from build123d import *
from build123d.topology import SkipClean

# Parameters (mm, degrees)
BOSS_EXTRUDE1_DEPTH   = 40
CUT_EXTRUDE4_DEPTH    = 149.681707012
FILLET1_R             = 20
CUT_EXTRUDE2_REACH    = 150.682
SKETCH3_R             = 19
M20_TAPPED_HOLE1_D    = 17.5
SKETCH8_R             = 15
CUT_EXTRUDE3_DEPTH    = 10
M6_TAPPED_HOLE1_D     = 5
M6_TAPPED_HOLE1_DEPTH = 17
M6_TAPPED_HOLE1_TIP   = 1.502151548
F_8_0MM_DOWEL_HOLE1_D = 8
CHAMFER1_SIZE         = 1


with BuildPart() as part:
    # Sketch1 → Boss-Extrude1 (new body)
    with BuildSketch(Plane(origin=(0, 0, 0), x_dir=(1, 0, 0), z_dir=(0, 1, 0))):
        with BuildLine():
            Line((-90, 0), (-90, 39.504902432))
            ThreePointArc((-90, 39.504902432), (-85.182396525, 94.862332258), (-30.561841884, 84.652075111))
            ThreePointArc((-30.561841884, 84.652075111), (0, 90), (30.561841884, 84.652075111))
            ThreePointArc((30.561841884, 84.652075111), (85.182396525, 94.862332258), (90, 39.504902432))
            Line((90, 39.504902432), (90, 0))
            ThreePointArc((90, 0), (0, -90), (-90, 0))
        make_face()
    extrude(amount=BOSS_EXTRUDE1_DEPTH)

    # Sketch2 → Cut-Extrude4 (cut, through all)
    with SkipClean():  # the faces are left unmerged after this step: merging them gives an invalid solid
        with BuildSketch(Plane(origin=(0, 0, 0), x_dir=(1, 0, 0), z_dir=(0, 1, 0))):
            with BuildLine():
                Line((-81.25, 32.524047358), (-62.5, 21.698729811))
                Line((-62.5, 21.698729811), (-62.5, 0))
                ThreePointArc((-62.5, 0), (0, -62.5), (62.5, 0))
                Line((62.5, 0), (62.5, 21.698729811))
                Line((62.5, 21.698729811), (81.25, 32.524047358))
                ThreePointArc((81.25, 32.524047358), (85.886934587, 35.68615872), (90, 39.504902432))
                Line((90, 39.504902432), (90, 0))
                ThreePointArc((90, 0), (0, -90), (-90, 0))
                Line((-90, 0), (-90, 39.504902432))
                ThreePointArc((-90, 39.504902432), (-85.886934587, 35.68615872), (-81.25, 32.524047358))
            make_face()
        extrude(amount=CUT_EXTRUDE4_DEPTH, mode=Mode.SUBTRACT)

    # Fillet1
    fillet1_edges = [part.edges().sort_by_distance(p)[0] for p in [
        (30.561841884, 20, -84.652075111),
        (-30.561841884, 20, -84.652075111),
        (-62.5, 20, -21.698729811),
        (62.5, 20, -21.698729811),
    ]]
    fillet(fillet1_edges, radius=FILLET1_R)

    # Sketch3 → Cut-Extrude2 (cut, up to next)
    with BuildSketch(Plane(origin=(0, 0, 0), x_dir=(1, 0, 0), z_dir=(0, 1, 0)), mode=Mode.PRIVATE) as cut_extrude2_sk1:
        with Locations(Location((-62.5, 65, 0), (0, 0, 270))):
            Circle(SKETCH3_R)
    cut_extrude2_tool1 = extrude(cut_extrude2_sk1.sketch, amount=CUT_EXTRUDE2_REACH, mode=Mode.PRIVATE) & part.part
    # Sketch3 → Cut-Extrude2 (cut, up to next)
    with BuildSketch(Plane(origin=(0, 0, 0), x_dir=(1, 0, 0), z_dir=(0, 1, 0)), mode=Mode.PRIVATE) as cut_extrude2_sk2:
        with Locations(Location((62.5, 65, 0), (0, 0, 270))):
            Circle(SKETCH3_R)
    cut_extrude2_tool2 = extrude(cut_extrude2_sk2.sketch, amount=CUT_EXTRUDE2_REACH, mode=Mode.PRIVATE) & part.part
    add(cut_extrude2_tool1.solids().sort_by_distance((-62.5, 0, -65))[0], mode=Mode.SUBTRACT)
    add(cut_extrude2_tool2.solids().sort_by_distance((62.5, 0, -65))[0], mode=Mode.SUBTRACT)

    # M20 Tapped Hole1 (through all)
    with Locations(Plane(origin=(0, 40, 0), x_dir=(1, 0, 0), z_dir=(0, 1, 0))):
        with Locations((0, 0)):
            Hole(M20_TAPPED_HOLE1_D / 2)

    # Sketch8 → Cut-Extrude3 (cut)
    with SkipClean():  # the faces are left unmerged after this step: merging them gives an invalid solid
        with BuildSketch(Plane.XZ):
            with Locations(Location((0, 0, 0), (0, 0, 270))):
                Circle(SKETCH8_R)
        extrude(amount=-CUT_EXTRUDE3_DEPTH, mode=Mode.SUBTRACT)

    # M6 Tapped Hole1
    with Locations(Plane(origin=(0, 0, 0), x_dir=(-1, 0, 0), z_dir=(0, -1, 0))):
        with Locations((-21.650635095, -12.237722392), (21.650635095, -12.5), (0, 25)):
            Hole(M6_TAPPED_HOLE1_D / 2, depth=M6_TAPPED_HOLE1_DEPTH)
            with Locations((0, 0, -(M6_TAPPED_HOLE1_DEPTH + M6_TAPPED_HOLE1_TIP / 2))):  # 118° drill point
                Cone(0, M6_TAPPED_HOLE1_D / 2, M6_TAPPED_HOLE1_TIP, mode=Mode.SUBTRACT)

    # Ø8.0mm Dowel Hole1 (through all)
    with Locations(Plane(origin=(0, 0, 0), x_dir=(-1, 0, 0), z_dir=(0, -1, 0))):
        with Locations((13.75, -23.815698604), (-13.75, 23.815698604)):
            Hole(F_8_0MM_DOWEL_HOLE1_D / 2)

    # Chamfer1
    chamfer1_edges = [part.edges().sort_by_distance(p)[0] for p in [
        (89.102687271, 40, -91.430040295),
        (0, 0, 62.5),
        (-62.5, 0, -5.075862213),
        (76.875, 0, -29.99813993),
        (0, 40, 62.5),
        (-62.5, 40, -5.075862213),
        (76.875, 40, -29.99813993),
        (62.5, 0, -5.075862213),
        (62.5, 40, -5.075862213),
        (-76.875, 0, -29.99813993),
        (-76.875, 40, -29.99813993),
        (0, 0, -90),
        (0, 40, -90),
        (-89.102687271, 0, -91.430040295),
        (-89.102687271, 40, -91.430040295),
        (65.179491924, 0, -20.151724427),
        (65.179491924, 40, -20.151724427),
        (-65.179491924, 0, -20.151724427),
        (-65.179491924, 40, -20.151724427),
        (28.863873105, 0, -88.103017476),
        (28.863873105, 40, -88.103017476),
        (-28.863873105, 0, -88.103017476),
        (-28.863873105, 40, -88.103017476),
        (89.102687271, 0, -91.430040295),
        (-62.5, 0, -84),
        (-62.5, 40, -84),
        (62.5, 0, -84),
        (62.5, 40, -84),
    ]]
    chamfer(chamfer1_edges, length=CHAMFER1_SIZE)


solid = part.part
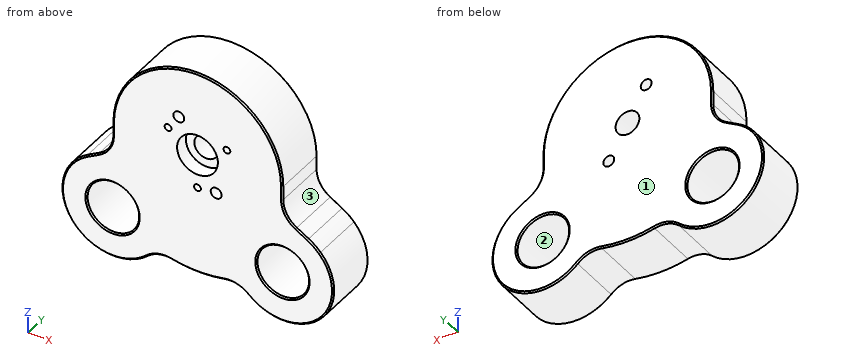
Source: CAD feature listing. Evaluate the final solid. Frame: model axes, mm. Face numbers are marked on the shaded views. Coordinates: 2 decimals unless noted, no trailing zeros. Loops run counter-clockwise (first coordinate to the right, second up) from the corner with the lowest first, then second, coordinate; pieces in that order, holes last. Notation, with made-up numbers: (46, -34.75) - (65, -34.75) arc R19 ccw to (65, -13.75) - close; hole circle Ø10 at (-23.75, 80.5). An arc over 180 degrees is marked (long way). Return JSON: item names as keys, results as strings.
Q1. Contact query for flat-ended pins moving along their axis: P1, Ø5, axis at x = 13.75, z = -23.82, coming from the -Y side; P2, Ø5, axis at y = 21.5, z = -13.5, coming from the +X side; P3, Ø12, axis at x = 71, y = 11.5, coming from the -Z side; P4, Ø2, axis at y = 34.5, z = 41.5, coming from the +X side. Output: stop coordinate, or through.
Results:
{"P1": "through", "P2": "x = 63.37", "P3": "z = -102.42", "P4": "x = 47.6"}
Q2. Material intervals for line 1 along X through (y, z) = (10, -65); line 2 along X through (y, z) = (4.5, -1); line 3 along X through (y, z) = (5, 12.5), sorted ascending.
Results:
{"line 1": "-100 to -81.5, -43.5 to 43.5, 81.5 to 100", "line 2": "-62.5 to -14.97, 14.97 to 62.5", "line 3": "-61.24 to -24.15, -19.15 to -8.29, 8.29 to 19.16, 24.14 to 61.24"}
Q3. Mould query, pull axis X, two halves, no side actions, for the marked faces 1, 2 and 3. Classes: released by +X, released by -X, zero draft, split by the parting line, or undercut.
Results:
{"face 1": "zero draft", "face 2": "undercut", "face 3": "released by +X"}
Q4. Section B-B, the plane y = 32. Give the number of separate pieces and of enclosed holes in the cut face, plus the area to 3 significant figures.
Results:
{"separate pieces": "1", "enclosed holes": "5", "area": "19,700 mm2"}
Q5. Section A-A, the plane z = -65. Return loops of the section in (x, y).
Results:
{"outline": "(-100, 1) - (-99, 0) - (-82.5, 0) - (-81.5, 1) - (-81.5, 39) - (-82.5, 40) - (-99, 40) - (-100, 39) - close; (-43.5, 1) - (-42.5, 0) - (42.5, 0) - (43.5, 1) - (43.5, 39) - (42.5, 40) - (-42.5, 40) - (-43.5, 39) - close; (81.5, 1) - (82.5, 0) - (99, 0) - (100, 1) - (100, 39) - (99, 40) - (82.5, 40) - (81.5, 39) - close"}
